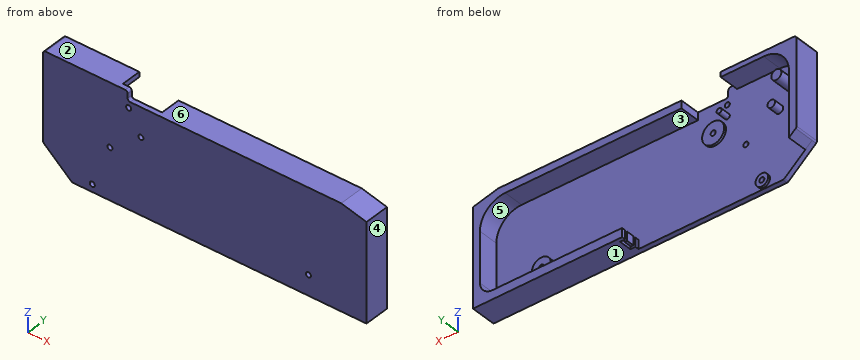
from build123d import *

# Parameters (mm, degrees)
SKETCH1_R               = 2
PRIMARY_DEPTH           = 4
SKETCH3_R               = 3
SKETCH3_R_2             = 2
STOP_EXT_DEPTH          = 8
FRONT_EXT_DEPTH         = 16
CUT_EXTRUDE1_START      = -7
SKETCH5_W               = 4
SKETCH5_H               = 2
CUT_EXTRUDE1_DEPTH      = 8
SKETCH6_W               = 2
SKETCH6_H               = 6
CUT_EXTRUDE2_DEPTH      = 3
SKETCH7_R               = 7.5
SKETCH7_R_2             = 2
SWINGYBIT_PIN_EXT_DEPTH = 6
SKETCH8_R               = 5
SKETCH8_R_2             = 2
SKETCH8_R_3             = 8.75
WHEEL_PIN_EXT_DEPTH     = 1.75
BOTTOM_EXT_DEPTH        = 16
FILLET1_R               = 2
SKETCH10_R              = 4
POST_EXT_DEPTH          = 16


with BuildPart() as part:
    # Sketch1 → Primary (new body)
    with BuildSketch(Plane(origin=(0, 0, 0), x_dir=(1, 0, 0), z_dir=(0, 1, 0))):
        Polygon((0, 0), (-23, -20), (-23, -90), (44, -90), (44, -82.5), (213, -82.5), (233, -77.5), (233, 0), align=None)
        with Locations((16, -6)):
            Circle(SKETCH1_R, mode=Mode.SUBTRACT)
        with Locations((30, -40.5)):
            Circle(SKETCH1_R, mode=Mode.SUBTRACT)
        with Locations((54.5, -59.5)):
            Circle(SKETCH1_R, mode=Mode.SUBTRACT)
        with Locations((44.75, -77.5)):
            Circle(SKETCH1_R, mode=Mode.SUBTRACT)
        with Locations((187, -16)):
            Circle(SKETCH1_R, mode=Mode.SUBTRACT)
    extrude(amount=PRIMARY_DEPTH)

    # Sketch3 → Stop Ext (add)
    with BuildSketch(Plane(origin=(0, 4, 0), x_dir=(1, 0, 0), z_dir=(0, 1, 0))):
        with Locations((3.5, -54.75)):
            Circle(SKETCH3_R)
        with Locations((44.75, -68.5)):
            Circle(SKETCH3_R_2)
    extrude(amount=STOP_EXT_DEPTH)

    # Sketch4 → Front Ext (add)
    with BuildSketch(Plane(origin=(0, 4, 0), x_dir=(1, 0, 0), z_dir=(0, 1, 0))):
        with BuildLine():
            Line((233, 0), (115, 0))
            Line((115, 0), (115, -7))
            Line((115, -7), (217.5, -7))
            ThreePointArc((217.5, -7), (224.571067812, -9.928932188), (227.5, -17))
            Line((227.5, -17), (227.5, -56.5))
            ThreePointArc((227.5, -56.5), (221.642135624, -70.642135624), (207.5, -76.5))
            Line((207.5, -76.5), (68, -76.5))
            Line((68, -76.5), (68, -82.5))
            Line((68, -82.5), (213, -82.5))
            Line((213, -82.5), (233, -77.5))
            Line((233, -77.5), (233, 0))
        make_face()
    extrude(amount=FRONT_EXT_DEPTH)

    # Sketch5 → Cut-Extrude1 (cut, through all)
    with BuildSketch(Plane(origin=(0, 0, 0), x_dir=(-1, 0, 0), z_dir=(0, 0, -1)).offset(CUT_EXTRUDE1_START)):
        with Locations((-117, 8)):
            Rectangle(SKETCH5_W, SKETCH5_H)
        with Locations((-117, 16)):
            Rectangle(SKETCH5_W, SKETCH5_H)
    extrude(amount=CUT_EXTRUDE1_DEPTH, mode=Mode.SUBTRACT)

    # Sketch6 → Cut-Extrude2 (cut)
    with BuildSketch(Plane(origin=(0, 0, 0), x_dir=(-1, 0, 0), z_dir=(0, 0, -1))):
        with Locations((-118, 12)):
            Rectangle(SKETCH6_W, SKETCH6_H)
    extrude(amount=-CUT_EXTRUDE2_DEPTH, mode=Mode.SUBTRACT)

    # Sketch7 → Swingybit_Pin Ext (add)
    with BuildSketch(Plane(origin=(0, 4, 0), x_dir=(1, 0, 0), z_dir=(0, 1, 0))):
        with Locations((187, -16)):
            Circle(SKETCH7_R)
        with Locations((187, -16)):
            Circle(SKETCH7_R_2, mode=Mode.SUBTRACT)
    extrude(amount=SWINGYBIT_PIN_EXT_DEPTH)

    # Sketch8 → Wheel_Pin Ext (add)
    with BuildSketch(Plane(origin=(0, 4, 0), x_dir=(1, 0, 0), z_dir=(0, 1, 0))):
        with Locations((16, -6)):
            Circle(SKETCH8_R)
        with Locations((16, -6)):
            Circle(SKETCH8_R_2, mode=Mode.SUBTRACT)
        with Locations((54.5, -59.5)):
            Circle(SKETCH8_R_3)
        with Locations((54.5, -59.5)):
            Circle(SKETCH8_R_2, mode=Mode.SUBTRACT)
    extrude(amount=WHEEL_PIN_EXT_DEPTH)

    # Sketch9 → Bottom Ext (add)
    with BuildSketch(Plane(origin=(0, 4, 0), x_dir=(1, 0, 0), z_dir=(0, 1, 0))):
        with BuildLine():
            Line((-23, -20), (-23, -86))
            Line((-23, -86), (-23, -90))
            Line((-23, -90), (37, -90))
            Line((37, -90), (37, -86))
            Line((37, -86), (3, -86))
            ThreePointArc((3, -86), (-11.142135624, -80.142135624), (-17, -66))
            Line((-17, -66), (-17, -14.782608696))
            Line((-17, -14.782608696), (-23, -20))
        make_face()
    extrude(amount=BOTTOM_EXT_DEPTH)

    # Fillet1
    fillet1_edges = [part.edges().sort_by_distance(p)[0] for p in [
        (44, 2, 82.5),
        (0, 2, 0),
        (-23, 10, 20),
        (-23, 10, 90),
        (44, 2, 90),
    ]]
    fillet(fillet1_edges, radius=FILLET1_R)

    # Sketch10 → Post Ext (add)
    with BuildSketch(Plane(origin=(0, 4, 0), x_dir=(1, 0, 0), z_dir=(0, 1, 0))):
        with Locations((-7, -67.5)):
            Circle(SKETCH10_R)
    extrude(amount=POST_EXT_DEPTH)


solid = part.part
The listing builds one solid part. Answer for the finished solid, in the listing's coordinates (mm). Face numbers are marked on the shaded views. A direction names the side the tool comes from. Round coordinates to 2 decimals unless told otherwise and drop trailing zeros. Order: outer loops, then holes, each group sorted by start corner. A loop starts at its lowest first (then second) coordinate and runs counter-clockwise, first axis right, second up. Notation, with made-up numbers: (88.5, 73.25) -> (134.5, 73.25) arc R29 ccw to (134.5, 105.25) -> close; hole circle Ø2 at (-22.75, 59.25). An arc over 180 degrees is marked (long way). One line per item, written item: value.
Item 1: Given P1, Ø7.5, axis at y = 12, z = 4, coming from the -X side; P2, Ø4.5, axis at y = 8, z = 88, coming from the +X side; P3, Ø3, axis at x = 3, z = 56, coming from the +Y side; P4, Ø2.5, axis at x = 30, z = 40.5, coming from the -Y side, each flat-ended and moving along its own axis, determine where each tip first touches the part or whether it passes through.
Taken from the geometry:
P1: stops at x = 115
P2: stops at x = 37
P3: stops at y = 12
P4: passes through
Item 2: For the marked faces 4, 5 and 6, determine the directions among +Z, -Z, +X, -X, +Y, -Y from which every point of the face is accessible in a straight line to the end or side of a thin tool.
Taken from the geometry:
face 4: +Z, -Z, +X, +Y, -Y
face 5: +Y
face 6: +Z, +X, +Y, -Y
Item 3: For a pull along Z with two mould halves and no side action, classify the marked faces 1, 2 and 3 as released by +Z, released by -Z, zero draft, split by the parting line, or undercut.
Taken from the geometry:
face 1: released by -Z
face 2: released by +Z
face 3: undercut
Item 4: Straight lines are drawn through the part: L1, parallel to Z at x = 187, y = 7.5; L2, parallel to Z at x = 161.5, y = 11; L3, parallel to Z at x = 16, y = 4.1. For each, find the intervals that lie inside material, in ascending order.
Taken from the geometry:
L1: z = 0 to 7, 8.5 to 14, 18 to 23.5, 76.5 to 82.5
L2: z = 0 to 7, 76.5 to 82.5
L3: z = 1 to 4, 8 to 11, 86 to 90
Item 5: Find section C-C, the plane x = 83. Give the vertices of the cut face in (y, z), then the cut area to 3 significant figures.
Taken from the geometry:
outline: (0, 0) -> (4, 0) -> (4, 76.5) -> (20, 76.5) -> (20, 82.5) -> (0, 82.5) -> close
area: 426 mm2
Item 6: Find section A-A, the plane z = 33. Give the vertices of the cut face in (x, y), then the cut area to 3 significant figures.
Taken from the geometry:
outline: (-23, 0) -> (233, 0) -> (233, 20) -> (227.5, 20) -> (227.5, 4) -> (-17, 4) -> (-17, 20) -> (-23, 20) -> close
area: 1,210 mm2
Item 7: Find section B-B, the plane x = 152.5. Give the vertices of the cut face in (y, z).
Taken from the geometry:
outline: (0, 0) -> (20, 0) -> (20, 7) -> (4, 7) -> (4, 76.5) -> (20, 76.5) -> (20, 82.5) -> (0, 82.5) -> close
